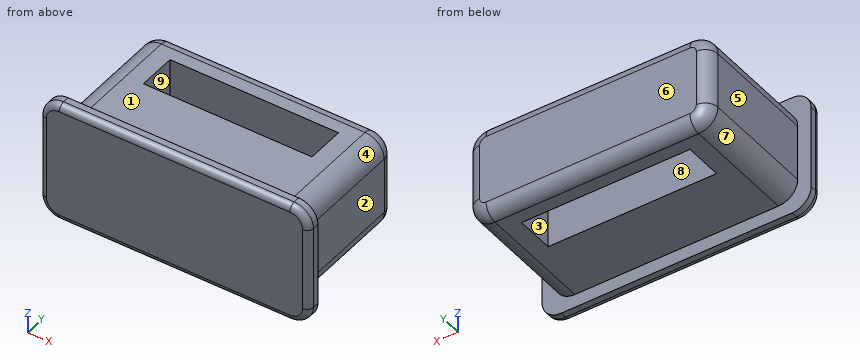
```python
from build123d import *

# Parameters (mm, degrees)
SKETCH1_W           = 42
SKETCH1_H           = 19
BOSS_EXTRUDE1_DEPTH = 2
FILLET1_R           = 3
FILLET2_R           = 1
SKETCH2_W           = 37.8
SKETCH2_H           = 14.8
BOSS_EXTRUDE2_DEPTH = 10
SKETCH3_W           = 5.75
SKETCH3_H           = 14.8
BOSS_EXTRUDE3_DEPTH = 10
SKETCH5_W           = 14.8
SKETCH5_H           = 4
BOSS_EXTRUDE4_DEPTH = 26.3
FILLET4_R           = 3
FILLET5_R           = 2


with BuildPart() as part:
    # Sketch1 → Boss-Extrude1 (new body)
    with BuildSketch(Plane(origin=(0, 0, 0), x_dir=(1, 0, 0), z_dir=(0, 1, 0))):
        with Locations((-35.747676634, 5.960595817)):
            Rectangle(SKETCH1_W, SKETCH1_H)
    extrude(amount=BOSS_EXTRUDE1_DEPTH)

    # Fillet1
    fillet1_edges = [part.edges().sort_by_distance(p)[0] for p in [
        (-56.747676634, 1, -15.460595817),
        (-14.747676634, 1, -15.460595817),
        (-14.747676634, 1, 3.539404183),
        (-56.747676634, 1, 3.539404183),
    ]]
    fillet(fillet1_edges, radius=FILLET1_R)

    # Fillet2
    fillet2_edges = [part.edges().sort_by_distance(p)[0] for p in [
        (-56.747676634, 0, -5.960595817),
        (-35.747676634, 0, -15.460595817),
        (-14.747676634, 0, -5.960595817),
        (-35.747676634, 0, 3.539404183),
        (-15.62635629, 0, 2.660724527),
        (-15.62635629, 0, -14.58191616),
        (-55.868996977, 0, 2.660724527),
        (-55.868996977, 0, -14.58191616),
    ]]
    fillet(fillet2_edges, radius=FILLET2_R)

    # Sketch2 → Boss-Extrude2 (add)
    with BuildSketch(Plane(origin=(0, 2, 0), x_dir=(1, 0, 0), z_dir=(0, 1, 0))):
        with Locations((-35.747676634, 5.960595817)):
            Rectangle(SKETCH2_W, SKETCH2_H)
    extrude(amount=BOSS_EXTRUDE2_DEPTH)

    # Sketch3 → Boss-Extrude3 (add)
    with BuildSketch(Plane(origin=(0, 12, 0), x_dir=(1, 0, 0), z_dir=(0, 1, 0))):
        with Locations((-19.722676634, 5.960595817)):
            Rectangle(SKETCH3_W, SKETCH3_H)
        with Locations((-51.772676634, 5.960595817)):
            Rectangle(SKETCH3_W, SKETCH3_H)
    extrude(amount=BOSS_EXTRUDE3_DEPTH)

    # Sketch5 → Boss-Extrude4 (add)
    with BuildSketch(Plane(origin=(-48.897676634, 0, 0), x_dir=(0, 0, -1), z_dir=(1, 0, 0))):
        with Locations((5.960595817, 20)):
            Rectangle(SKETCH5_W, SKETCH5_H)
    extrude(amount=BOSS_EXTRUDE4_DEPTH)

    # Fillet4
    fillet4_edges = [part.edges().sort_by_distance(p)[0] for p in [
        (-54.647676634, 12, -13.360595817),
        (-54.647676634, 12, 1.439404183),
        (-16.847676634, 12, 1.439404183),
        (-16.847676634, 12, -13.360595817),
    ]]
    fillet(fillet4_edges, radius=FILLET4_R)

    # Fillet5
    fillet5_edges = [part.edges().sort_by_distance(p)[0] for p in [
        (-35.747676634, 22, -13.360595817),
        (-16.847676634, 22, -5.960595817),
        (-35.747676634, 22, 1.439404183),
        (-54.647676634, 22, -5.960595817),
        (-53.768996977, 22, 0.560724527),
        (-53.768996977, 22, -12.48191616),
        (-17.72635629, 22, 0.560724527),
        (-17.72635629, 22, -12.48191616),
    ]]
    fillet(fillet5_edges, radius=FILLET5_R)


solid = part.part
```
Geometry check sheet. Reference: the model listing, model coordinates, mm. Face numbers are marked on the shaded views. A direction names the side the tool comes from. Round coordinates to 2 decimals unless told otherwise and drop trailing zeros. Loops run counter-clockwise (first coordinate to the right, second up) from the corner with the lowest first, then second, coordinate; pieces in that order, holes last. Notation, with made-up numbers: (37.25, 32.25) - (76.25, 32.25) arc R15 ccw to (76.25, 40.25) - close; hole circle Ø6 at (48.25, 59.5). An arc over 180 degrees is marked (long way). Write each question's results on one line, items separated by ' | '. Start each with the question number.
Q1. Cross-section at C-C on z = -3.25. Enter the section's corners in (x, y), and give its area (3 significant figures).
Q2. Cross-section at D-D on y = 11. Enter the section's corners in (x, z), and give its area (3 significant figures).
Q3. Gauge pin test, flat ends, axial feed: P1, Ø5, axis at x = -22, y = 10, coming from the -Z side; P2, Ø2, axis at y = 4.5, z = -9.5, coming from the -X side; P3, Ø1.8, axis at y = 14, z = -3, coming from the +X side. Record the tip position at first contact, or that the pin passes through.
Q4. Access from +Z, -Z, +X, -X, +Y, -Y to the whole of each face (thin tool, end or side, straight path). Record for the marked faces 1, 2, 3, 4 and 5.
Q5. Cross-section at B-B on y = 14.75. Enter the section's corners in (x, z).
Q6. Release check for a two-part mould opening along Y. For the marked faces 6, 7, 8 and 9 record: +Y half, -Y half, draft (parallel to the pull), parting line (faces both ways), or undercut.
Q7. Cross-section at A-A on x = -29.5. Enter the section's corners in (y, z).
Q8. Thickness scan on line 1 (Y direction, x = -35.5, z = -11.25); line 2 (X direction, y = 13.75, z = -2.5); line 3 (Y direction, x = -39.5, z = -13). Record the ranges inside material, lowest first. Write a range as [from, to].
Answers below:
1) outline: (-56.75, 1) arc R1 ccw to (-55.75, 0) - (-15.75, 0) arc R1 ccw to (-14.75, 1) - (-14.75, 2) - (-16.85, 2) - (-16.85, 20) arc R2 ccw to (-18.85, 22) - (-52.65, 22) arc R2 ccw to (-54.65, 20) - (-54.65, 2) - (-56.75, 2) - close; hole (-48.9, 12) - (-22.6, 12) - (-22.6, 18) - (-48.9, 18) - close | area: 680 mm²
2) outline: (-54.65, -10.36) arc R3 ccw to (-51.65, -13.36) - (-19.85, -13.36) arc R3 ccw to (-16.85, -10.36) - (-16.85, -1.56) arc R3 ccw to (-19.85, 1.44) - (-51.65, 1.44) arc R3 ccw to (-54.65, -1.56) - close | area: 552 mm²
3) P1: stops at z = -13.36 | P2: stops at x = -54.65 | P3: stops at x = -16.85
4) face 1: +Z, +X, -X, +Y | face 2: +Z, -Z, +X, +Y | face 3: +Z, -Z | face 4: +Z, +X, +Y | face 5: +Z, -Z, -X, +Y
5) outline: (-54.65, -10.36) arc R3 ccw to (-51.65, -13.36) - (-48.9, -13.36) - (-48.9, 1.44) - (-51.65, 1.44) arc R3 ccw to (-54.65, -1.56) - close; (-22.6, -13.36) - (-19.85, -13.36) arc R3 ccw to (-16.85, -10.36) - (-16.85, -1.56) arc R3 ccw to (-19.85, 1.44) - (-22.6, 1.44) - close
6) face 6: +Y half | face 7: draft | face 8: undercut | face 9: undercut
7) outline: (0, -14.46) arc R1 ccw to (1, -15.46) - (2, -15.46) - (2, -13.36) - (12, -13.36) - (12, 1.44) - (2, 1.44) - (2, 3.54) - (1, 3.54) arc R1 ccw to (0, 2.54) - close; (18, -13.36) - (20, -13.36) arc R2 ccw to (22, -11.36) - (22, -0.56) arc R2 ccw to (20, 1.44) - (18, 1.44) - close
8) line 1: y = [0, 12], [18, 22] | line 2: x = [-54.65, -48.9], [-22.6, -16.85] | line 3: y = [0, 12], [18, 21.15]
